Source: CAD feature listing. Evaluate the final solid. Frame: model axes, mm. Face numbers are marked on the shaded views. Give positions to 0.01 mm unless a question says otherwise; leave off trailing zeros. Loops run counter-clockwise (first coordinate to the right, second up) from the corner with the lowest first, then second, coordinate; pieces in that order, holes last. Notation, with made-up numbers: (78.25, 61) -> (91.25, 61) arc R18 ccw to (91.25, 92) -> close; hole circle Ø3 at (8, 36.5). An arc over 180 degrees is marked (long way). Put each result on its own line as item: value.
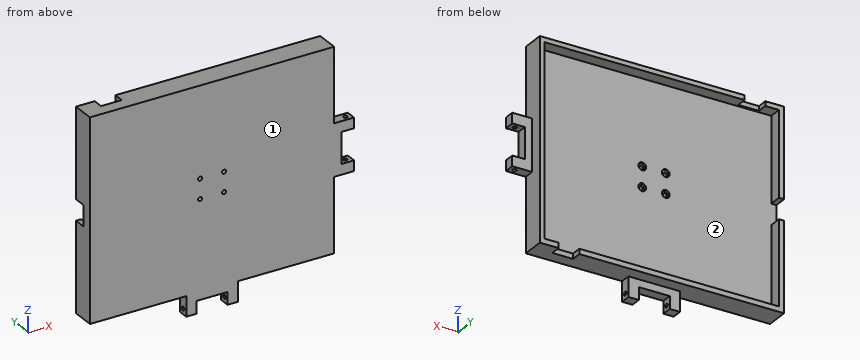
```python
from build123d import *

# Parameters (mm, degrees)
SKETCH2_W           = 236.5
SKETCH2_H           = 193
SKETCH2_W_2         = 227
SKETCH2_H_2         = 183.5
BOSS_EXTRUDE1_DEPTH = 12.1
SKETCH3_W           = 236.5
SKETCH3_H           = 193
BOSS_EXTRUDE2_DEPTH = 10
SKETCH4_W           = 10
SKETCH4_H           = 10
CUT_EXTRUDE1_DEPTH  = 5
SKETCH7_W           = 20
SKETCH7_H           = 10
CUT_EXTRUDE2_DEPTH  = 5
SKETCH8_W           = 20
SKETCH8_H           = 10
CUT_EXTRUDE3_DEPTH  = 5
SKETCH14_W          = 25
SKETCH14_H          = 10
BOSS_EXTRUDE6_DEPTH = 19.25
SKETCH18_W          = 12.25
SKETCH18_H          = 30
CUT_EXTRUDE7_DEPTH  = 11
SKETCH19_R          = 1.925
CUT_EXTRUDE8_DEPTH  = 122.5
SKETCH21_R          = 1.925
CUT_EXTRUDE9_DEPTH  = 23.1
SKETCH22_R          = 3.75
SKETCH22_R_2        = 1.925
CUT_EXTRUDE10_DEPTH = 2.4
SKETCH27_W          = 25
SKETCH27_H          = 10
BOSS_EXTRUDE7_DEPTH = 19.25
SKETCH28_W          = 30
SKETCH28_H          = 12
CUT_EXTRUDE11_DEPTH = 19.25
SKETCH31_R          = 1.925
CUT_EXTRUDE12_DEPTH = 144.25
SKETCH32_W          = 20
SKETCH32_H          = 12.1
CUT_EXTRUDE14_DEPTH = 6


with BuildPart() as part:
    # Sketch2 → Boss-Extrude1 (new body)
    with BuildSketch(Plane(origin=(0, 0, 0), x_dir=(1, 0, 0), z_dir=(0, 1, 0))):
        with Locations((113.25, -91.5)):
            Rectangle(SKETCH2_W, SKETCH2_H)
        with Locations((113.5, -91.75)):
            Rectangle(SKETCH2_W_2, SKETCH2_H_2, mode=Mode.SUBTRACT)
    extrude(amount=BOSS_EXTRUDE1_DEPTH)

    # Sketch3 → Boss-Extrude2 (add)
    with BuildSketch(Plane.XZ):
        with Locations((113.25, 91.5)):
            Rectangle(SKETCH3_W, SKETCH3_H)
    extrude(amount=BOSS_EXTRUDE2_DEPTH)

    # Sketch4 → Cut-Extrude1 (cut)
    with BuildSketch(Plane.ZY.offset(5)):
        with Locations((96.5, 7.1)):
            Rectangle(SKETCH4_W, SKETCH4_H)
        with Locations((86.5, 7.1)):
            Rectangle(SKETCH4_W, SKETCH4_H)
    extrude(amount=-CUT_EXTRUDE1_DEPTH, mode=Mode.SUBTRACT)

    # Sketch7 → Cut-Extrude2 (cut)
    with BuildSketch(Plane.XY.offset(188)):
        with Locations((23.25, 7.1)):
            Rectangle(SKETCH7_W, SKETCH7_H)
    extrude(amount=-CUT_EXTRUDE2_DEPTH, mode=Mode.SUBTRACT)

    # Sketch8 → Cut-Extrude3 (cut)
    with BuildSketch(Plane(origin=(0, 0, -5), x_dir=(-1, 0, 0), z_dir=(0, 0, -1))):
        with Locations((-203.25, 7.1)):
            Rectangle(SKETCH8_W, SKETCH8_H)
    extrude(amount=-CUT_EXTRUDE3_DEPTH, mode=Mode.SUBTRACT)

    # Sketch14 → Boss-Extrude6 (add)
    with BuildSketch(Plane(origin=(231.5, 0, 0), x_dir=(0, 0, -1), z_dir=(1, 0, 0))):
        with Locations((-104, -5)):
            Rectangle(SKETCH14_W, SKETCH14_H)
        with Locations((-79, -5)):
            Rectangle(SKETCH14_W, SKETCH14_H)
    extrude(amount=BOSS_EXTRUDE6_DEPTH)

    # Sketch18 → Cut-Extrude7 (cut, through all)
    with BuildSketch(Plane(origin=(0, 0, 0), x_dir=(1, 0, 0), z_dir=(0, 1, 0))):
        with Locations((244.625, -91.5)):
            Rectangle(SKETCH18_W, SKETCH18_H)
    extrude(amount=-CUT_EXTRUDE7_DEPTH, mode=Mode.SUBTRACT)

    # Sketch19 → Cut-Extrude8 (cut, through all)
    with BuildSketch(Plane.XY.offset(116.5)):
        with Locations((245.378954084, -5)):
            Circle(SKETCH19_R)
    extrude(amount=-CUT_EXTRUDE8_DEPTH, mode=Mode.SUBTRACT)

    # Sketch21 → Cut-Extrude9 (cut, through all)
    with BuildSketch(Plane.XZ.offset(10)):
        with Locations((124.871391666, 82.016158176)):
            Circle(SKETCH21_R)
        with Locations((124.871391666, 100.983841824)):
            Circle(SKETCH21_R)
        with Locations((101.628608334, 100.983841824)):
            Circle(SKETCH21_R)
        with Locations((101.628608334, 82.016158176)):
            Circle(SKETCH21_R)
    extrude(amount=-CUT_EXTRUDE9_DEPTH, mode=Mode.SUBTRACT)

    # Sketch22 → Cut-Extrude10 (cut)
    with BuildSketch(Plane(origin=(0, 0, 0), x_dir=(1, 0, 0), z_dir=(0, 1, 0))):
        with Locations((102.128608334, -82.016158176)):
            Circle(SKETCH22_R)
        with Locations((101.628608334, -82.016158176)):
            Circle(SKETCH22_R_2, mode=Mode.SUBTRACT)
        with Locations((124.871391666, -82.016158176)):
            Circle(SKETCH22_R)
        with Locations((124.871391666, -82.016158176)):
            Circle(SKETCH22_R_2, mode=Mode.SUBTRACT)
        with Locations((124.871391666, -101.483841824)):
            Circle(SKETCH22_R)
        with Locations((124.871391666, -100.983841824)):
            Circle(SKETCH22_R_2, mode=Mode.SUBTRACT)
        with Locations((102.128608334, -101.483841824)):
            Circle(SKETCH22_R)
        with Locations((101.628608334, -100.983841824)):
            Circle(SKETCH22_R_2, mode=Mode.SUBTRACT)
    extrude(amount=-CUT_EXTRUDE10_DEPTH, mode=Mode.SUBTRACT)

    # Sketch27 → Boss-Extrude7 (add)
    with BuildSketch(Plane(origin=(0, 0, -5), x_dir=(-1, 0, 0), z_dir=(0, 0, -1))):
        with Locations((-125.75, -5)):
            Rectangle(SKETCH27_W, SKETCH27_H)
        with Locations((-100.75, -5)):
            Rectangle(SKETCH27_W, SKETCH27_H)
    extrude(amount=BOSS_EXTRUDE7_DEPTH)

    # Sketch28 → Cut-Extrude11 (cut)
    with BuildSketch(Plane(origin=(0, 0, 0), x_dir=(1, 0, 0), z_dir=(0, 1, 0))):
        with Locations((113.25, 18.25)):
            Rectangle(SKETCH28_W, SKETCH28_H)
    extrude(amount=-CUT_EXTRUDE11_DEPTH, mode=Mode.SUBTRACT)

    # Sketch31 → Cut-Extrude12 (cut, through all)
    with BuildSketch(Plane(origin=(138.25, 0, 0), x_dir=(0, 0, -1), z_dir=(1, 0, 0))):
        with Locations((18.88, -5)):
            Circle(SKETCH31_R)
    extrude(amount=-CUT_EXTRUDE12_DEPTH, mode=Mode.SUBTRACT)

    # Sketch32 → Cut-Extrude14 (cut, through all)
    with BuildSketch(Plane(origin=(0, 0, 0), x_dir=(0, 0, -1), z_dir=(1, 0, 0))):
        with Locations((-91.5, 6.05)):
            Rectangle(SKETCH32_W, SKETCH32_H)
    extrude(amount=-CUT_EXTRUDE14_DEPTH, mode=Mode.SUBTRACT)


solid = part.part
```
(1) Section A-A on y = 5. Return loops of the section in (x, z), then the cut area to 3 significant figures.
Calculated:
outline: (-5, -5) -> (193.25, -5) -> (193.25, 0) -> (0, 0) -> (0, 81.5) -> (-5, 81.5) -> close; (-5, 101.5) -> (0, 101.5) -> (0, 183.5) -> (13.25, 183.5) -> (13.25, 188) -> (-5, 188) -> close; (33.25, 183.5) -> (227, 183.5) -> (227, 0) -> (213.25, 0) -> (213.25, -5) -> (231.5, -5) -> (231.5, 188) -> (33.25, 188) -> close
area: 3,700 mm²
(2) First-contact query: P1, Ø5, axis at x = 236.5, y = -7, coming from the -Z side; P2, Ø8.5, axis at x = 124.87, z = 82.02, coming from the +Y side; P3, Ø2.5, axis at x = 101.63, z = 100.98, coming from the -Y side; P4, Ø6, axis at y = 8.5, z = 89.5, coming from the -X side. Flat tips, straight axial feed; report the tip coordinate or a pass-through.
Calculated:
P1: stops at z = 66.5
P2: stops at y = 0
P3: passes through
P4: stops at x = 227
(3) Line query: probe 1 along Z at (x, y) = (156.5, 10.5); probe 2 along X at (y, z) = (3.25, 123); probe 3 along Y at (x, z) = (234.5, 79). Output: solid intervals per line, ascending. Write a range as from..to.
Calculated:
probe 1: z = -5..0, 183.5..188
probe 2: x = -5..0, 227..231.5
probe 3: y = -10..0
(4) Draft query along Z for the marked faces 1 and 2. Return one class per face: released by +Z, released by -Z, zero draft, split by the parting line, or undercut.
Calculated:
face 1: zero draft
face 2: undercut
(5) Section B-B on x = 91. Return loops of the section in (y, z) (3 decimals), then the cut area to 3 significant figures.
Calculated:
outline: (-10, -24.25) -> (0, -24.25) -> (0, -5) -> (12.1, -5) -> (12.1, 0) -> (0, 0) -> (0, 183.5) -> (12.1, 183.5) -> (12.1, 188) -> (-10, 188) -> close; hole circle Ø3.85 at (-5, -18.88)
area: 2,230 mm²
(6) Section C-C on z = 142. Return loops of the section in (x, y).
Calculated:
outline: (-5, -10) -> (231.5, -10) -> (231.5, 12.1) -> (227, 12.1) -> (227, 0) -> (0, 0) -> (0, 12.1) -> (-5, 12.1) -> close
(7) Section D-D on x = 21.5. Return loops of the section in (y, z).
Calculated:
outline: (-10, -5) -> (12.1, -5) -> (12.1, 0) -> (0, 0) -> (0, 183.5) -> (2.1, 183.5) -> (2.1, 188) -> (-10, 188) -> close
